Read the model definition and answer for the solid it produces. Units are mm, in the model's axes. A direction names the side the tool comes from. Give positions to 0.01 mm unless a question says otherwise; leave off trailing zeros. Loops run counter-clockwise (first coordinate to the right, second up) from the corner with the lowest first, then second, coordinate; pieces in that order, holes last. Notation, with made-up numbers: (56, 77.5) - (109, 77.5) arc R29 cw to (109, 103.5) - close; hole circle Ø6 at (-11, 16). An arc over 180 degrees is marked (long way). Use a Markdown table: item, result. Add a question column.
Item 1: Which of the six approach directions +Z, -Z, +X, -X, +Y, -Y give full straight-line access (tool end or side, diameter ignored) to faces 4 (the face through (0, 4, 15)), 5 (the face through (7.758, 7.798, 17.874)), 6 (the face through (0, -16, 22)), 7 (the face through (-19, 0, 19)), 8 (the face through (20, 0, 16))?
Item 2: A cutting plane is placed at D-D (z = 3.25). Determine the outline of the cut face in (x, y), plus the area to 3 significant figures.
Item 3: Consider probe 1 along X at (y, z) = (9, 23.5); probe 2 along X at (y, z) = (12, 12.75); probe 3 along X at (y, z) = (0.5, 12.75). Determine where each line is inside the solid, lowest interval first. Write a range as [from, to].
Item 4: Each of these flat-tipped pins is pushed along its axis until it touches: P1, Ø8, axis at x = 5, y = -15.5, coming from the +Z side; P2, Ø8, axis at x = -18, y = 6.5, coming from the +Z side; P3, Ø2.5, axis at y = 1, z = 22, coming from the +X side. Where does it stop, or does it pass through?
Item 5: A cutting plane is placed at A-A (z = 9.75). Determine the outline of the cut face in (x, y).
Item 6: A cutting plane is placed at B-B (y = -21). Determine the outline of the cut face in (x, z), plus the area to 3 significant figures.
Item 7: A cutting plane is placed at C-C (z = 19.75). Determine the outline of the cut face in (x, y).
Item 8: For a pull along X with two mould halves and no side action, classify faces 1 (the face through (-17.542, 16.085, 4.437)), 2 (the face through (-19.2, 0.2, 16)), 3 (the face through (7, -9, 9)) as +X half, -X half, draft (parallel to the pull), parting line (faces both ways), or undercut.
from build123d import *

# Parameters (mm, degrees)
SKETCH1_R        = 23.8
STEP1_DEPTH      = 9
SKETCH2_R        = 22
STEP2_DEPTH      = 7
SKETCH3_R        = 19
STEP3_DEPTH      = 6
SKETCH4_R        = 15
STEP4_DEPTH      = 5
LOBED_TOP_DEPTH  = 3
FLUTES_DEPTH     = 18
SKETCH7_R        = 4
BORE_DEPTH       = 30
SKETCH8_W        = 1.2
SKETCH8_H        = 9
BORE_FLATS_DEPTH = 30


with BuildPart() as part:
    # Sketch1 → Step1 (new body)
    with BuildSketch(Plane.XY):
        Circle(SKETCH1_R)
    extrude(amount=STEP1_DEPTH)

    # Sketch2 → Step2 (add)
    with BuildSketch(Plane.XY.offset(9)):
        Circle(SKETCH2_R)
    extrude(amount=STEP2_DEPTH)

    # Sketch3 → Step3 (add)
    with BuildSketch(Plane.XY.offset(16)):
        Circle(SKETCH3_R)
    extrude(amount=STEP3_DEPTH)

    # Sketch4 → Step4 (add)
    with BuildSketch(Plane.XY.offset(22)):
        Circle(SKETCH4_R)
    extrude(amount=STEP4_DEPTH)

    # Sketch5 → Lobed_top (add)
    with BuildSketch(Plane.XY.offset(27)):
        Polygon((12.5, 0), (12.405234104, 0.813082), (12.127403917, 1.596603015), (11.68528529, 2.32434776), (11.108147002, 2.976419019), (10.432933463, 3.541503697), (9.700735091, 4.01817604), (8.952908293, 4.415085774), (8.227241336, 4.75), (7.554555327, 5.047792488), (6.956081779, 5.33758928), (6.441875004, 5.649372756), (6.01040764, 6.01040764), (5.649372756, 6.441875004), (5.33758928, 6.956081779), (5.047792488, 7.554555327), (4.75, 8.227241336), (4.415085774, 8.952908293), (4.01817604, 9.700735091), (3.541503697, 10.432933463), (2.976419019, 11.108147002), (2.32434776, 11.68528529), (1.596603015, 12.127403917), (0.813082, 12.405234104), (0, 12.5), (-0.813082, 12.405234104), (-1.596603015, 12.127403917), (-2.32434776, 11.68528529), (-2.976419019, 11.108147002), (-3.541503697, 10.432933463), (-4.01817604, 9.700735091), (-4.415085774, 8.952908293), (-4.75, 8.227241336), (-5.047792488, 7.554555327), (-5.33758928, 6.956081779), (-5.649372756, 6.441875004), (-6.01040764, 6.01040764), (-6.441875004, 5.649372756), (-6.956081779, 5.33758928), (-7.554555327, 5.047792488), (-8.227241336, 4.75), (-8.952908293, 4.415085774), (-9.700735091, 4.01817604), (-10.432933463, 3.541503697), (-11.108147002, 2.976419019), (-11.68528529, 2.32434776), (-12.127403917, 1.596603015), (-12.405234104, 0.813082), (-12.5, 0), (-12.405234104, -0.813082), (-12.127403917, -1.596603015), (-11.68528529, -2.32434776), (-11.108147002, -2.976419019), (-10.432933463, -3.541503697), (-9.700735091, -4.01817604), (-8.952908293, -4.415085774), (-8.227241336, -4.75), (-7.554555327, -5.047792488), (-6.956081779, -5.33758928), (-6.441875004, -5.649372756), (-6.01040764, -6.01040764), (-5.649372756, -6.441875004), (-5.33758928, -6.956081779), (-5.047792488, -7.554555327), (-4.75, -8.227241336), (-4.415085774, -8.952908293), (-4.01817604, -9.700735091), (-3.541503697, -10.432933463), (-2.976419019, -11.108147002), (-2.32434776, -11.68528529), (-1.596603015, -12.127403917), (-0.813082, -12.405234104), (0, -12.5), (0.813082, -12.405234104), (1.596603015, -12.127403917), (2.32434776, -11.68528529), (2.976419019, -11.108147002), (3.541503697, -10.432933463), (4.01817604, -9.700735091), (4.415085774, -8.952908293), (4.75, -8.227241336), (5.047792488, -7.554555327), (5.33758928, -6.956081779), (5.649372756, -6.441875004), (6.01040764, -6.01040764), (6.441875004, -5.649372756), (6.956081779, -5.33758928), (7.554555327, -5.047792488), (8.227241336, -4.75), (8.952908293, -4.415085774), (9.700735091, -4.01817604), (10.432933463, -3.541503697), (11.108147002, -2.976419019), (11.68528529, -2.32434776), (12.127403917, -1.596603015), (12.405234104, -0.813082), align=None)
    extrude(amount=LOBED_TOP_DEPTH)

    # Sketch6 → Flutes (cut)
    with BuildSketch(Plane.XY.offset(9)):
        Polygon((9.192388155, 6.363961031), (19.657568517, 16.829141392), (16.829141392, 19.657568517), (6.363961031, 9.192388155), align=None)
        Polygon((-6.363961031, 9.192388155), (-16.829141392, 19.657568517), (-19.657568517, 16.829141392), (-9.192388155, 6.363961031), align=None)
        Polygon((-9.192388155, -6.363961031), (-19.657568517, -16.829141392), (-16.829141392, -19.657568517), (-6.363961031, -9.192388155), align=None)
        Polygon((6.363961031, -9.192388155), (16.829141392, -19.657568517), (19.657568517, -16.829141392), (9.192388155, -6.363961031), align=None)
    extrude(amount=FLUTES_DEPTH, mode=Mode.SUBTRACT)

    # Sketch7 → Bore (cut)
    with BuildSketch(Plane.XY):
        Circle(SKETCH7_R)
    extrude(amount=BORE_DEPTH, mode=Mode.SUBTRACT)

    # Sketch8 → Bore_flats (add)
    with BuildSketch(Plane.XY):
        with Locations((3.85, 0)):
            Rectangle(SKETCH8_W, SKETCH8_H)
        with Locations((-3.85, 0)):
            Rectangle(SKETCH8_W, SKETCH8_H)
    extrude(amount=BORE_FLATS_DEPTH)


solid = part.part
Geometry says:
| question | item | result |
|---|---|---|
| 1 | face 4 | +Z, -Z |
| 1 | face 5 | +Z |
| 1 | face 6 | +Z, -Y |
| 1 | face 7 | +Z, -X |
| 1 | face 8 | +Z, +X |
| 2 | outline | circle Ø47.6 at (0, 0); hole (-3.25, -2.33) arc R4 ccw to (3.25, -2.33) - (3.25, 2.33) arc R4 ccw to (-3.25, 2.33) - close |
| 2 | area | 1,730 mm² |
| 3 | probe 1 | [-12, -11.83], [-6.56, 6.56], [11.83, 12] |
| 3 | probe 2 | [-18.44, -14.83], [-9.17, 9.17], [14.83, 18.44] |
| 3 | probe 3 | [-21.99, -3.25], [3.25, 21.99] |
| 4 | P1 | z = 27 |
| 4 | P2 | z = 22 |
| 4 | P3 | x = 19 |
| 5 | outline | (-16.91, -14.08) - (-9.19, -6.36) - (-6.36, -9.19) - (-14.08, -16.91) arc R22 ccw to (14.08, -16.91) - (6.36, -9.19) - (9.19, -6.36) - (16.91, -14.08) arc R22 ccw to (16.91, 14.08) - (9.19, 6.36) - (6.36, 9.19) - (14.08, 16.91) arc R22 ccw to (-14.08, 16.91) - (-6.36, 9.19) - (-9.19, 6.36) - (-16.91, 14.08) arc R22 ccw to start; hole (-3.25, -2.33) arc R4 ccw to (3.25, -2.33) - (3.25, 2.33) arc R4 ccw to (-3.25, 2.33) - close |
| 6 | outline | (-11.2, 0) - (11.2, 0) - (11.2, 9) - (6.56, 9) - (6.56, 16) - (-6.56, 16) - (-6.56, 9) - (-11.2, 9) - close |
| 6 | area | 293 mm² |
| 7 | outline | (-14.77, -11.95) - (-9.19, -6.36) - (-6.36, -9.19) - (-11.95, -14.77) arc R19 ccw to (11.95, -14.77) - (6.36, -9.19) - (9.19, -6.36) - (14.77, -11.95) arc R19 ccw to (14.77, 11.95) - (9.19, 6.36) - (6.36, 9.19) - (11.95, 14.77) arc R19 ccw to (-11.95, 14.77) - (-6.36, 9.19) - (-9.19, 6.36) - (-14.77, 11.95) arc R19 ccw to start; hole (-3.25, -2.33) arc R4 ccw to (3.25, -2.33) - (3.25, 2.33) arc R4 ccw to (-3.25, 2.33) - close |
| 8 | face 1 | parting line |
| 8 | face 2 | draft |
| 8 | face 3 | undercut |
